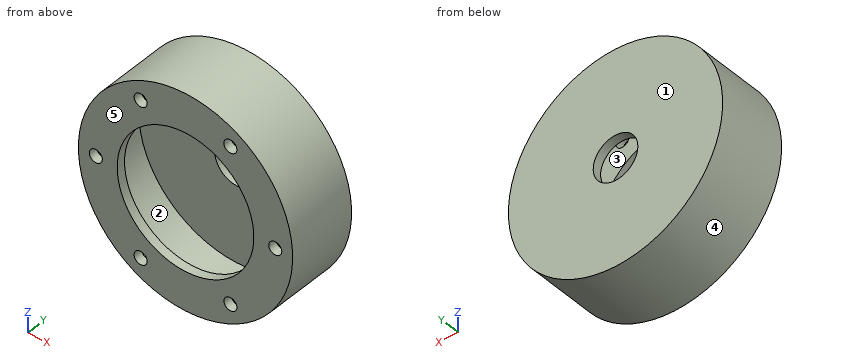
from build123d import *

# Parameters (mm, degrees)
SKETCH1_W          = 139.7
SKETCH1_H          = 12.7
SKETCH1_W_2        = 107.95
SKETCH1_H_2        = 12.744604202
CUT_EXTRUDE3_REACH = 240.273
SKETCH5_R          = 97.248113747
SKETCH5_R_2        = 9.267203016


with BuildPart() as part:
    # Sketch1 → Revolve1 (revolve)
    with BuildSketch(Plane.XY, mode=Mode.PRIVATE) as revolve1_sk:
        Polygon((-152.4, 0), (-139.7, 0), (-139.7, 12.7), (-139.7, 88.855395798), (-139.7, 101.6), (-152.4, 101.6), align=None)
        with Locations((-69.85, 6.35)):
            Rectangle(SKETCH1_W, SKETCH1_H)
        with Locations((-85.725, 95.227697899)):
            Rectangle(SKETCH1_W_2, SKETCH1_H_2)
    revolve(revolve1_sk.sketch.rotate(Axis((0, 50.8, 0), (0, 1, 0)), 270), axis=Axis((0, 50.8, 0), (0, 1, 0)))

    # Sketch5 → Cut-Extrude3 (cut, up to next)
    with BuildSketch(Plane.XZ, mode=Mode.PRIVATE) as cut_extrude3_sk1:
        with Locations(Location((0, 0, 0), (0, 0, 270))):
            Circle(SKETCH5_R)
    cut_extrude3_tool1 = extrude(cut_extrude3_sk1.sketch, amount=-CUT_EXTRUDE3_REACH, mode=Mode.PRIVATE) & part.part
    # Sketch5 → Cut-Extrude3 (cut, up to next)
    with BuildSketch(Plane.XZ, mode=Mode.PRIVATE) as cut_extrude3_sk2:
        with Locations(Location((127.67505098, 0, 0), (0, 0, 270))):
            Circle(SKETCH5_R_2)
    cut_extrude3_tool2 = extrude(cut_extrude3_sk2.sketch, amount=-CUT_EXTRUDE3_REACH, mode=Mode.PRIVATE) & part.part
    # Sketch5 → Cut-Extrude3 (cut, up to next)
    with BuildSketch(Plane.XZ, mode=Mode.PRIVATE) as cut_extrude3_sk3:
        with Locations(Location((63.83752549, -110.569837578, 0), (0, 0, 270))):
            Circle(SKETCH5_R_2)
    cut_extrude3_tool3 = extrude(cut_extrude3_sk3.sketch, amount=-CUT_EXTRUDE3_REACH, mode=Mode.PRIVATE) & part.part
    # Sketch5 → Cut-Extrude3 (cut, up to next)
    with BuildSketch(Plane.XZ, mode=Mode.PRIVATE) as cut_extrude3_sk4:
        with Locations(Location((-63.83752549, -110.569837578, 0), (0, 0, 270))):
            Circle(SKETCH5_R_2)
    cut_extrude3_tool4 = extrude(cut_extrude3_sk4.sketch, amount=-CUT_EXTRUDE3_REACH, mode=Mode.PRIVATE) & part.part
    # Sketch5 → Cut-Extrude3 (cut, up to next)
    with BuildSketch(Plane.XZ, mode=Mode.PRIVATE) as cut_extrude3_sk5:
        with Locations(Location((-127.67505098, 0, 0), (0, 0, 270))):
            Circle(SKETCH5_R_2)
    cut_extrude3_tool5 = extrude(cut_extrude3_sk5.sketch, amount=-CUT_EXTRUDE3_REACH, mode=Mode.PRIVATE) & part.part
    # Sketch5 → Cut-Extrude3 (cut, up to next)
    with BuildSketch(Plane.XZ, mode=Mode.PRIVATE) as cut_extrude3_sk6:
        with Locations(Location((-63.83752549, 110.569837578, 0), (0, 0, 270))):
            Circle(SKETCH5_R_2)
    cut_extrude3_tool6 = extrude(cut_extrude3_sk6.sketch, amount=-CUT_EXTRUDE3_REACH, mode=Mode.PRIVATE) & part.part
    # Sketch5 → Cut-Extrude3 (cut, up to next)
    with BuildSketch(Plane.XZ, mode=Mode.PRIVATE) as cut_extrude3_sk7:
        with Locations(Location((63.83752549, 110.569837578, 0), (0, 0, 270))):
            Circle(SKETCH5_R_2)
    cut_extrude3_tool7 = extrude(cut_extrude3_sk7.sketch, amount=-CUT_EXTRUDE3_REACH, mode=Mode.PRIVATE) & part.part
    add(cut_extrude3_tool1.solids().sort_by_distance((0, 0, 0))[0], mode=Mode.SUBTRACT)
    add(cut_extrude3_tool2.solids().sort_by_distance((127.675051, 0, 0))[0], mode=Mode.SUBTRACT)
    add(cut_extrude3_tool3.solids().sort_by_distance((63.837525, 0, -110.569838))[0], mode=Mode.SUBTRACT)
    add(cut_extrude3_tool4.solids().sort_by_distance((-63.837525, 0, -110.569838))[0], mode=Mode.SUBTRACT)
    add(cut_extrude3_tool5.solids().sort_by_distance((-127.675051, 0, 0))[0], mode=Mode.SUBTRACT)
    add(cut_extrude3_tool6.solids().sort_by_distance((-63.837525, 0, 110.569838))[0], mode=Mode.SUBTRACT)
    add(cut_extrude3_tool7.solids().sort_by_distance((63.837525, 0, 110.569838))[0], mode=Mode.SUBTRACT)


solid = part.part
Geometry check sheet. Reference: the model listing, model coordinates, mm. Face numbers are marked on the shaded views. A direction names the side the tool comes from. Give positions to 0.01 mm unless a question says otherwise; leave off trailing zeros. Order: outer loops, then holes, each group sorted by start corner. A loop starts at its lowest first (then second) coordinate and runs counter-clockwise, first axis right, second up. Notation, with made-up numbers: M -28.5,35 L -6.5,35 A26 cw -6.5,52 Z; hole C 73.5,51.25 d2. An arc over 180 degrees is marked long. Use a Markdown table: item, result.
Item 1: Section check C-C (y = 65.5). Record the cut outline in (x, z).
Answers follow:
| item | result |
|---|---|
| outline | C 0,0 d304.8; hole C 0,0 d279.4 |
Item 2: Draft check along Z on the marked faces 3, 4 and 5. Enter one of: +Z half, -Z half, draft (parallel to the pull), parting line (faces both ways), or undercut.
Answers follow:
| item | result |
|---|---|
| face 3 | undercut |
| face 4 | parting line |
| face 5 | draft |
Item 3: Section check B-B (z = 0). Record the cut outline in (x, y), and give its area (3 significant figures).
Answers follow:
| item | result |
|---|---|
| outline | M -152.4,0 L -136.94,0 L -136.94,12.7 L -139.7,12.7 L -139.7,88.86 L -31.75,88.86 L -31.75,101.6 L -152.4,101.6 Z; M -118.41,0 L -97.25,0 L -97.25,12.7 L -118.41,12.7 Z; M 31.75,88.86 L 139.7,88.86 L 139.7,12.7 L 136.94,12.7 L 136.94,0 L 152.4,0 L 152.4,101.6 L 31.75,101.6 Z; M 97.25,0 L 118.41,0 L 118.41,12.7 L 97.25,12.7 Z |
| area | 5,940 mm2 |
Item 4: Depth check by flat-ended pin: P1, Ø11, axis at x = -63.84, z = 110.57, coming from the -Y side; P2, Ø12, axis at y = 23, z = -77, coming from the -X side; P3, Ø10, axis at x = -0.5, y = 66, coming from the -Z side; P4, Ø10, axis at y = 81, z = -30.5, coming from the +X side. Enter the tip coordinate at first touch or a pass-through.
Answers follow:
| item | result |
|---|---|
| P1 | stops at y = 88.86 |
| P2 | stops at x = -134.85 |
| P3 | stops at z = -152.4 |
| P4 | stops at x = 150.25 |
Item 5: Section check A-A (x = 0). Record the cut outline in (y, z), and give its area (3 significant figures).
Answers follow:
| item | result |
|---|---|
| outline | M 0,-152.4 L 101.6,-152.4 L 101.6,-31.75 L 88.86,-31.75 L 88.86,-139.7 L 12.7,-139.7 L 12.7,-97.25 L 0,-97.25 Z; M 0,97.25 L 12.7,97.25 L 12.7,139.7 L 88.86,139.7 L 88.86,31.75 L 101.6,31.75 L 101.6,152.4 L 0,152.4 Z |
| area | 6,410 mm2 |
Item 6: Tool access check on the marked faces 1 and 2. Record the directions out of +Z, -Z, +X, -X, +Y, -Y that give a thin tool (end or side, any length) a straight path to the whole face; none if there is none.
Answers follow:
| item | result |
|---|---|
| face 1 | +Z, -Z, +X, -X, +Y |
| face 2 | none |
Item 7: Section check D-D (z = 113.5). Record the cut outline in (x, y), and give its area (3 significant figures).
Answers follow:
| item | result |
|---|---|
| outline | M -101.7,0 L -72.63,0 L -72.63,12.7 L -81.45,12.7 L -81.45,88.86 L 81.45,88.86 L 81.45,12.7 L 72.63,12.7 L 72.63,0 L 101.7,0 L 101.7,101.6 L -101.7,101.6 Z; M -55.05,0 L 55.05,0 L 55.05,12.7 L -55.05,12.7 Z |
| area | 7,810 mm2 |
Item 8: Material ranges on line 1 along X through (y, z) = (6, 0); line 2 along Y through (x, z) = (-102, 92); line 3 along Y through (x, z) = (62, -69.5), recorded low to high.
Answers follow:
| item | result |
|---|---|
| line 1 | x = -152.4 to -136.94, -118.41 to -97.25, 97.25 to 118.41, 136.94 to 152.4 |
| line 2 | y = 0 to 12.7, 88.86 to 101.6 |
| line 3 | y = 88.86 to 101.6 |
